Geometry: see drawing. Coordinates: mm, zero at the bounding-box minimum. Coordinates: 2 decimals unless noted, no trailing zeros. Write each loop counter-clockwise with the first axis right and the second up, starting at its lowest first coordinate (ties: lowest second). Pieces come first, ordered by that corner, then holes. Notation, with made-up numbers: (55, 10.5) -> (87, 10.5) arc R30 ccw to (87, 36.5) -> close; hole circle Ø1 at (77, 35.25). An arc over 180 degrees is marked (long way). Answer as a JSON object with one key per item and string values. Group by question number.
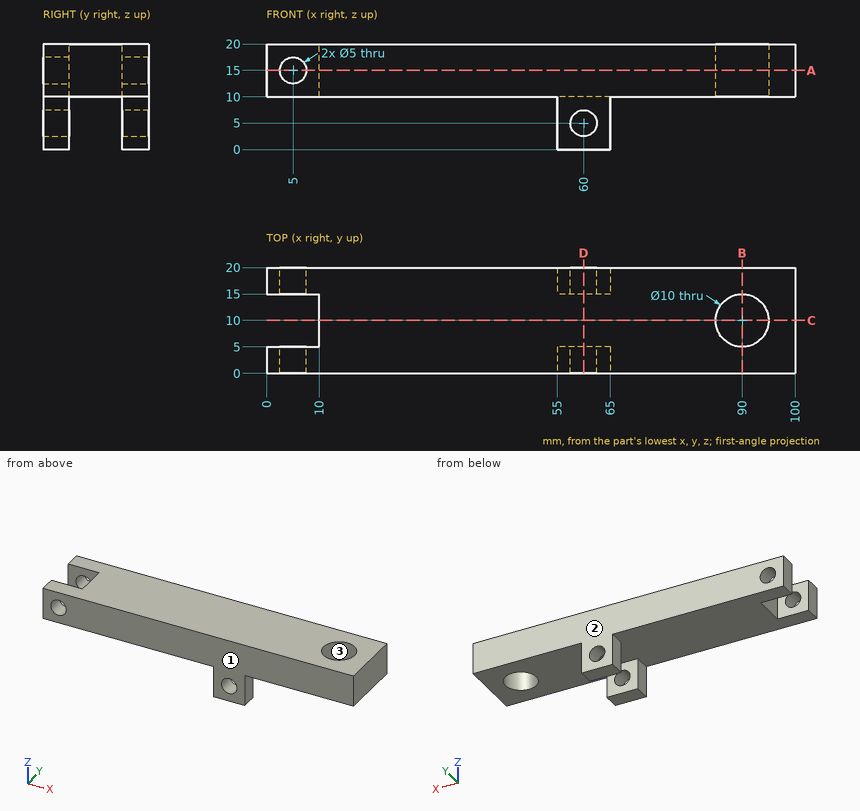
Item 1: Section C-C on y = 10. Output: boundary loops of the cut face in (x, z).
Item 2: Section B-B on x = 90. Output: boundary loops of the cut face in (y, z).
Item 3: Section A-A on z = 15. Output: boundary loops of the cut face in (x, y), then the cut area to 3 significant figures.
Item 4: Mould query, pull axis Y, two halves, no side actions, for the marked faces 1, 2 and 3. Classes: +Y half, -Y half, draft (parallel to the pull), parting line (faces both ways), or undercut.
Item 5: Contact query for flat-ended pins moving along their axis: pin 1 (10 mm diameter, centred on x = 37, y = 15, fed in from -Z); pin 2 (6 mm diameter, centred on x = 5, z = 15, fed in from +Y); pin 3 (4 mm diameter, centred on y = 1.5, z = 5.5, fed in from +X); pin 4 (4 mm diameter, centred on x = 60, z = 5, fed in from -Y). Output: stop coordinate, or through.
Item 6: Section D-D on x = 60. Output: boundary loops of the cut face in (y, z), then the cut area to 3 significant figures.
Item 7: Ray query, L1, parallel to X at y = 18.35, z = 5; L2, parallel to Y at x = 90, z = 14.25; L3, parallel to X at y = 17.15, z = 15. Return the intervals inside material, ascending. Write a range as [from, to].
Answer sheet:
{
 "1": {"outline": "(10, 10) -> (85, 10) -> (85, 20) -> (10, 20) -> close; (95, 10) -> (100, 10) -> (100, 20) -> (95, 20) -> close"},
 "2": {"outline": "(0, 10) -> (5, 10) -> (5, 20) -> (0, 20) -> close; (15, 10) -> (20, 10) -> (20, 20) -> (15, 20) -> close"},
 "3": {"outline": "(0, 0) -> (2.5, 0) -> (2.5, 5) -> (0, 5) -> close; (0, 15) -> (2.5, 15) -> (2.5, 20) -> (0, 20) -> close; (7.5, 0) -> (100, 0) -> (100, 20) -> (7.5, 20) -> (7.5, 15) -> (10, 15) -> (10, 5) -> (7.5, 5) -> close; hole circle Ø10 at (90, 10)", "area": "1,770 mm^2"},
 "4": {"face 1": "-Y half", "face 2": "+Y half", "face 3": "undercut"},
 "5": {"pin 1": "stops at z = 10", "pin 2": "stops at y = 20", "pin 3": "stops at x = 65", "pin 4": "passes through"},
 "6": {"outline": "(0, 0) -> (5, 0) -> (5, 2.5) -> (0, 2.5) -> close; (0, 7.5) -> (5, 7.5) -> (5, 10) -> (15, 10) -> (15, 7.5) -> (20, 7.5) -> (20, 20) -> (0, 20) -> close; (15, 0) -> (20, 0) -> (20, 2.5) -> (15, 2.5) -> close", "area": "250 mm^2"},
 "7": {"L1": "x = [55, 57.5], [62.5, 65]", "L2": "y = [0, 5], [15, 20]", "L3": "x = [0, 2.5], [7.5, 100]"}
}
